Design review of the part built by this model. Coordinates are the model's own, in mm. Face numbers are marked on the shaded views. Round coordinates to 2 decimals unless told otherwise and drop trailing zeros. Order: outer loops, then holes, each group sorted by start corner. A loop starts at its lowest first (then second) coordinate and runs counter-clockwise, first axis right, second up. Notation, with made-up numbers: M 29.5,-10 L 59.5,-10 A26 ccw 59.5,9 Z; hole C 48,67.5 d7. An arc over 180 degrees is marked long. Write each question's results on one line, items separated by ' | '. Start each with the question number.
Item 1: Clearance check with flat-ended pins moving along their axes: pin 1 (1.5 mm diameter, centred on y = 2, z = -28.5, fed in from -X); pin 2 (1 mm diameter, centred on y = 1.5, z = -24, fed in from -X). State where each tip first meets the part, or that it passes through.
Item 2: Take a section at C-C, the plane x = 35.5. Write out the cut boundary in (y, z).
Item 3: Wall thickness on line 1 (X direction, y = 2.3, z = -1.5) (3 decimals); line 2 (X direction, y = 3.3, z = -31); line 3 (Z direction, x = 22.5, y = 1.3): over which ranges is each line inside the solid? List them lowest first. Write a range as [from, to].
Item 4: Take a section at D-D, the plane z = -11. Write out the cut boundary in (x, y).
Item 5: The part is to be moulded in two halves that separate along Z. For the marked faces 1, 2, 3 and 4, say which applies: +Z half, -Z half, draft (parallel to the pull), parting line (faces both ways), or undercut.
Item 6: Take a section at A-A, the plane z = -2.5. Write out the cut boundary in (x, y) (3 decimals), plus the area to 3 significant figures.
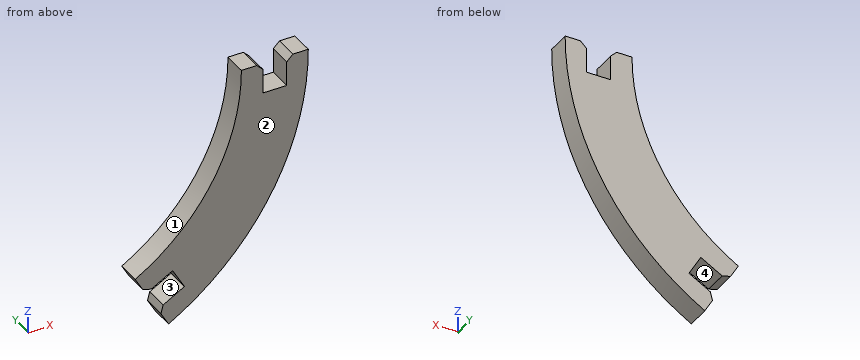
```python
from build123d import *

# Parameters (mm, degrees)
BOSS_EXTRUDE1_DEPTH = 3.85
CHAMFER1_SIZE       = 1


with BuildPart() as part:
    # Sketch1 → Boss-Extrude1 (new body)
    with BuildSketch(Plane(origin=(0, 0, 0), x_dir=(1, 0, 0), z_dir=(0, 1, 0))):
        with BuildLine():
            Line((37.975, 0), (37.975, 5))
            Line((37.975, 5), (41.825, 5))
            Line((41.825, 5), (41.825, 0))
            Line((41.825, 0), (45.325, 0))
            ThreePointArc((45.325, 0), (39.252601427, 22.6625), (22.6625, 39.252601427))
            Line((22.6625, 39.252601427), (20.9125, 36.221512513))
            Line((20.9125, 36.221512513), (25.242627019, 33.721512513))
            Line((25.242627019, 33.721512513), (23.317627019, 30.387314709))
            Line((23.317627019, 30.387314709), (18.9875, 32.887314709))
            Line((18.9875, 32.887314709), (17.2375, 29.856225795))
            ThreePointArc((17.2375, 29.856225795), (29.856225795, 17.2375), (34.475, 0))
            Line((34.475, 0), (37.975, 0))
        make_face()
    extrude(amount=BOSS_EXTRUDE1_DEPTH)

    # Chamfer1
    chamfer1_edges = [part.edges().sort_by_distance(p)[0] for p in [
        (18.9875, 1.925, -32.887314709),
        (20.9125, 1.925, -36.221512513),
        (41.825, 1.925, 0),
        (37.975, 1.925, 0),
    ]]
    chamfer(chamfer1_edges, length=CHAMFER1_SIZE)


solid = part.part
```
Results list:
1) pin 1: x = 18.25 | pin 2: x = 24.25
2) outline: M 0,-28.18 L 3.85,-28.18 L 3.85,0 L 0,0 Z
3) line 1: [34.442, 37.975], [41.825, 45.3] | line 2: [17.9, 22.26], [23.67, 33.07] | line 3: [-38.97, -35.3], [-30.86, -26.12]
4) outline: M 32.67,0 L 43.97,0 L 43.97,3.85 L 32.67,3.85 Z
5) face 1: +Z half | face 2: draft | face 3: undercut | face 4: undercut
6) outline: M 34.384,0 L 37.975,0 L 37.975,3.85 L 34.384,3.85 Z; M 41.825,0 L 45.256,0 L 45.256,3.85 L 41.825,3.85 Z | area: 27.0 mm²
